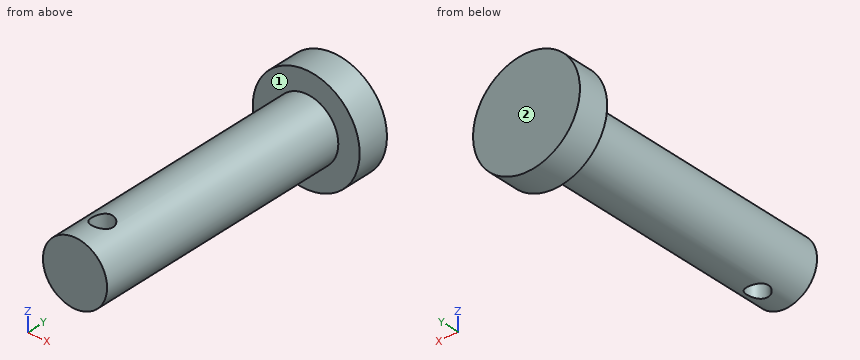
from build123d import *

# Parameters (mm, degrees)
F0_R     = 2.5
F1_DEPTH = 1.5
F2_R     = 1.5
F3_DEPTH = 12.7
F5_R     = 0.5
F6_DEPTH = 4.001


with BuildPart() as f1:
    # F0 (on Front) → F1 (new body)
    with BuildSketch(Plane.XZ):
        Circle(F0_R)
    extrude(amount=F1_DEPTH)

    # F2 (on face) → F3 (join)
    with BuildSketch(Plane.XZ.offset(1.5)):
        Circle(F2_R)
    extrude(amount=F3_DEPTH)

    # F5 (on offset) → F6 (cut, through all)
    with BuildSketch(Plane.XY.offset(1.5)):
        with Locations((0, -12.7)):
            Circle(F5_R)
    extrude(amount=-F6_DEPTH, mode=Mode.SUBTRACT)


solid = f1.part
Can you work these out from the model? Positions are in its coordinate system, mm. Face numbers are marked on the shaded views. A direction names the side the tool comes from. Round coordinates to 2 decimals unless told otherwise and drop trailing zeros. Order: outer loops, then holes, each group sorted by start corner. A loop starts at its lowest first (then second) coordinate and runs counter-clockwise, first axis right, second up. Notation, with made-up numbers: (-26.75, 49) - (20.25, 49) arc R23 cw to (20.25, 73) - close; hole circle Ø3 at (30.25, 3). An arc over 180 degrees is marked (long way). Answer in a Markdown table with one row per item.
(1) Suppose I cut it at B-B, the plane x = 0. Please give me the cut outline in (y, z).
From the geometry:
| item | result |
|---|---|
| outline | (-14.2, -1.5) - (-13.2, -1.5) - (-13.2, 1.5) - (-14.2, 1.5) - close; (-12.2, -1.5) - (-1.5, -1.5) - (-1.5, -2.5) - (0, -2.5) - (0, 2.5) - (-1.5, 2.5) - (-1.5, 1.5) - (-12.2, 1.5) - close |
(2) Suppose I cut it at A-A, the plane z = 0. Please give me the cut outline in (x, y).
From the geometry:
| item | result |
|---|---|
| outline | (-2.5, -1.5) - (-1.5, -1.5) - (-1.5, -14.2) - (1.5, -14.2) - (1.5, -1.5) - (2.5, -1.5) - (2.5, 0) - (-2.5, 0) - close; hole circle Ø1 at (0, -12.7) |
(3) Please list where these lines run through material, in increasing order: L1, parallel to Y at x = 0, z = -0.55; L2, parallel to X at y = -12.7, z = 0.05; L3, parallel to X at y = -12.7, z = -0.9. Write a range as from..to.
From the geometry:
| item | result |
|---|---|
| L1 | y = -14.2..-13.2, -12.2..0 |
| L2 | x = -1.5..-0.5, 0.5..1.5 |
| L3 | x = -1.2..-0.5, 0.5..1.2 |
(4) Suppose I cut it at C-C, the plane y = -2.5. Please give me the cut outline in (x, z), plus the area to 3 significant figures.
From the geometry:
| item | result |
|---|---|
| outline | circle Ø3 at (0, 0) |
| area | 7.07 mm2 |
(5) Suppose I cut it at D-D, the plane x = -0.9. Please give me the cut outline in (y, z).
From the geometry:
| item | result |
|---|---|
| outline | (-14.2, -1.2) - (-1.5, -1.2) - (-1.5, -2.33) - (0, -2.33) - (0, 2.33) - (-1.5, 2.33) - (-1.5, 1.2) - (-14.2, 1.2) - close |
(6) For P1, Ø3, axis at x = -1.5, y = -8.5, coming from the -Z side; P2, Ø3, axis at y = -5.5, z = -0.5, coming from the -X side; P3, Ø1, axis at x = 0.5, y = -4.5, coming from the +Z side, each with a flat end and sliding along its axis, tell me the tip position at first contact or that it passes through.
From the geometry:
| item | result |
|---|---|
| P1 | stops at z = -1.5 |
| P2 | stops at x = -1.5 |
| P3 | stops at z = 1.5 |
(7) Which directions (+Z, -Z, +X, -X, +Y, -Y) give clear straight access to the entire face, cutting with the end or side of a thin tool? Please do the marked faces 1 and 2.
From the geometry:
| item | result |
|---|---|
| face 1 | -Y |
| face 2 | +Z, -Z, +X, -X, +Y |
